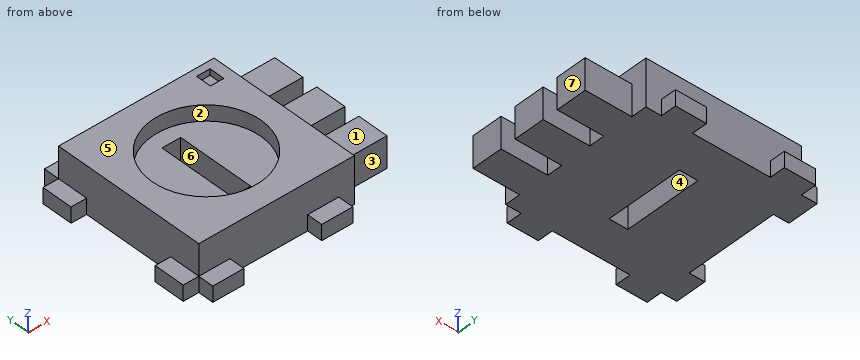
```python
from build123d import *

# Parameters (mm, degrees)
F0_W      = 50
F0_H      = 50
F1_DEPTH  = 15
F2_W      = 6
F2_H      = 25
F3_DEPTH  = 25
F4_W      = 10
F4_H      = 10
F5_DEPTH  = 30
F6_W      = 50
F6_H      = 20
F7_DEPTH  = 30
F9_DEPTH  = 50
F10_DEPTH = 5
F11_R     = 17.5
F11_W     = 6
F11_H     = 25
F12_DEPTH = 5
F11_W_2   = 25
F11_H_2   = 5.1409158856
F11_W_3   = 5
F11_H_3   = 5
F11_H_4   = 30
F13_DEPTH = 25
F14_W     = 6
F14_H     = 6
F15_DEPTH = 20
F16_DEPTH = 15
F11_W_4   = 4.3280106038
F11_H_5   = 4.9385428429
F17_DEPTH = 2
F18_W     = 60
F18_H     = 62
F19_DEPTH = 25
F20_SCALE = 1.6
F21_DEPTH = 4
F22_DEPTH = 4


with BuildPart() as f1:
    # F0 (on Top) → F1 (new body)
    with BuildSketch(Plane.XY):
        Rectangle(F0_W, F0_H)
    extrude(amount=F1_DEPTH)

    # F2 (on face) → F3 (cut)
    with BuildSketch(Plane.XY.offset(15)):
        Rectangle(F2_W, F2_H)
    extrude(amount=-F3_DEPTH, mode=Mode.SUBTRACT)

    # F4 (on face) → F5 (join)
    with BuildSketch(Plane.YZ.offset(25)):
        with Locations((0, 7.5)):
            Rectangle(F4_W, F4_H)
        with Locations((-15, 7.5)):
            Rectangle(F4_W, F4_H)
        with Locations((15, 7.5)):
            Rectangle(F4_W, F4_H)
    extrude(amount=F5_DEPTH)

    # F6 (on face) → F7 (join)
    with BuildSketch(Plane.YZ.offset(55)):
        with Locations((0, 7.5)):
            Rectangle(F6_W, F6_H)
    extrude(amount=F7_DEPTH)

    # F8 (on face) → F9 (cut)
    with BuildSketch(Plane(origin=(0, 25, 0), x_dir=(-1, 0, 0), z_dir=(0, 1, 0))):
        Polygon((-85, -2.5), (-70, 17.5), (-85, 17.5), align=None)
    extrude(amount=-F9_DEPTH, mode=Mode.SUBTRACT)

    # F0 (on Top) → F10 (join)
    with BuildSketch(Plane.XY):
        Polygon((-25, -25), (-25, 25), (25, 25), (25, 30), (-30, 30), (-30, -30), (25, -30), (25, -25), align=None)
    extrude(amount=F10_DEPTH)

    # F11 (on face) → F12 (cut)
    with BuildSketch(Plane.XY.offset(15)):
        Circle(F11_R)
        Rectangle(F11_W, F11_H, mode=Mode.SUBTRACT)
    extrude(amount=-F12_DEPTH, mode=Mode.SUBTRACT)

    # F11 (on face) → F13 (cut)
    with BuildSketch(Plane.XY.offset(15)):
        with Locations((-2.5, -27.5704579428)):
            Rectangle(F11_W_2, F11_H_2)
        with Locations((-27.5, -27.5704579428)):
            Rectangle(F11_W_3, F11_H_2)
        with Locations((22.5, -27.5704579428)):
            Rectangle(F11_W_3, F11_H_2)
        with Locations((22.5, 27.5)):
            Rectangle(F11_W_3, F11_H_3)
        with Locations((-2.5, 27.5)):
            Rectangle(F11_W_2, F11_H_3)
        with Locations((-27.5, 27.5)):
            Rectangle(F11_W_3, F11_H_3)
        with Locations((-27.5, 0)):
            Rectangle(F11_W_3, F11_H_4)
    extrude(amount=-F13_DEPTH, mode=Mode.SUBTRACT)

    # F14 (on face) → F15 (join)
    with BuildSketch(Plane.XY.offset(17.5)):
        with Locations((67, 28)):
            Rectangle(F14_W, F14_H)
        with Locations((67, -28)):
            Rectangle(F14_W, F14_H)
    extrude(amount=-F15_DEPTH)

    # F14 (on face) → F16 (cut)
    with BuildSketch(Plane.XY.offset(17.5)):
        with Locations((67, -28)):
            Rectangle(F14_W, F14_H)
        with Locations((67, 28)):
            Rectangle(F14_W, F14_H)
    extrude(amount=-F16_DEPTH, mode=Mode.SUBTRACT)

    # F11 (on face) → F17 (cut)
    with BuildSketch(Plane.XY.offset(15)):
        with Locations((19.372981973, 20.1403833926)):
            Rectangle(F11_W_4, F11_H_5)
    extrude(amount=-F17_DEPTH, mode=Mode.SUBTRACT)

    # F18 (on face) → F19 (cut)
    with BuildSketch(Plane.XY.offset(17.5)):
        with Locations((70, 0)):
            Rectangle(F18_W, F18_H)
    extrude(amount=-F19_DEPTH, mode=Mode.SUBTRACT)


with BuildPart() as f1_1:
    # F20: moved
    add(f1.part.scale(F20_SCALE).moved(Location((0, 0, -9))))

    # F21 (add): faces of the model
    f21_faces = [f1_1.faces().sort_by_distance(p)[0] for p in [
        (52, 24, -5),
        (52, 0, -5),
        (52, -24, -5),
    ]]
    extrude(f21_faces, amount=F21_DEPTH)

    # F22 (cut): faces of the model
    f22_faces = [f1_1.faces().sort_by_distance(p)[0] for p in [
        (52, 24, 11),
        (52, 0, 11),
        (52, -24, 11),
    ]]
    extrude(f22_faces, amount=-F22_DEPTH, mode=Mode.SUBTRACT)


solid = f1_1.part
```
Geometry check sheet. Reference: the model listing, model coordinates, mm. Face numbers are marked on the shaded views. A direction names the side the tool comes from. Round coordinates to 2 decimals unless told otherwise and drop trailing zeros. Order: outer loops, then holes, each group sorted by start corner. A loop starts at its lowest first (then second) coordinate and runs counter-clockwise, first axis right, second up. Notation, with made-up numbers: (62, -25) -> (77, -25) arc R20 ccw to (77, -2) -> close; hole circle Ø11 at (-14, -35.75). An arc over 180 degrees is marked (long way). Return JSON: item names as keys, results as strings. Group by question number.
Q1. Section check B-B, the plane z = 0.75. Record the boundary of the cut face in (x, y), plus the area to 3 significant figures.
Q2. Release check for a two-part mould opening along X. For the marked faces 5, 6 and 7 record: released by +X, released by -X, zero draft, split by the parting line, or undercut.
Q3. Tool access check on the marked faces 1, 2, 3 and 4. Record the directions out of +Z, -Z, +X, -X, +Y, -Y that give a thin tool (end or side, any length) a straight path to the whole face; none if there is none.
Q4. Material ranges on probe 1 along Y at (x, z) = (0, 8.75); probe 2 along Y at (x, z) = (-40.5, -3); probe 3 along X at (y, z) = (3.5, -6.5), recorded low to high. Write a range as from..to.
Q5. Section check D-D, the plane x = 49. Record the boundary of the cut face in (y, z), plus the area to 3 significant figures.
Q6. Gauge pin test, flat ends, axial feed: pin 1 (8 mm diameter, centred on x = 54.5, z = -3.5, fed in from +Y); pin 2 (3.5 mm diameter, centred on y = 31, z = 13.5, fed in from -X); pin 3 (6 mm diameter, centred on x = 13.5, z = 4, fed in from +Y). Record the tip position at first contact, or that the pin passes through.
Q7. Section check A-A, the plane y = 0. Record the boundary of the cut face in (x, z).
Q8. Section check C-C, the plane x = 0. Record the boundary of the cut face in (y, z).
Numbers:
{
 "1": {"outline": "(-40, -40) -> (40, -40) -> (40, -32) -> (64, -32) -> (64, -16) -> (40, -16) -> (40, -8) -> (64, -8) -> (64, 8) -> (40, 8) -> (40, 16) -> (64, 16) -> (64, 32) -> (40, 32) -> (40, 40) -> (-40, 40) -> close; hole (-4.8, -20) -> (4.8, -20) -> (4.8, 20) -> (-4.8, 20) -> close", "area": "7,170 mm^2"},
 "2": {"face 5": "zero draft", "face 6": "undercut", "face 7": "released by +X"},
 "3": {"face 1": "+Z, +X, +Y, -Y", "face 2": "+Z", "face 3": "+Z, -Z, +X, -Y", "face 4": "+Z, -Z"},
 "4": {"probe 1": "-40..-28, 28..40", "probe 2": "-40..-24, 24..40", "probe 3": "-40..-4.8, 4.8..64"},
 "5": {"outline": "(-32, -9) -> (-16, -9) -> (-16, 7) -> (-32, 7) -> close; (-8, -9) -> (8, -9) -> (8, 7) -> (-8, 7) -> close; (16, -9) -> (32, -9) -> (32, 7) -> (16, 7) -> close", "area": "768 mm^2"},
 "6": {"pin 1": "y = 32", "pin 2": "x = -40", "pin 3": "y = 40"},
 "7": {"outline": "(-40, -9) -> (-4.8, -9) -> (-4.8, 7) -> (-28, 7) -> (-28, 15) -> (-40, 15) -> close; (4.8, -9) -> (64, -9) -> (64, 7) -> (40, 7) -> (40, 15) -> (28, 15) -> (28, 7) -> (4.8, 7) -> close"},
 "8": {"outline": "(-40, -9) -> (-20, -9) -> (-20, 7) -> (-28, 7) -> (-28, 15) -> (-40, 15) -> close; (20, -9) -> (40, -9) -> (40, 15) -> (28, 15) -> (28, 7) -> (20, 7) -> close"}
}
